Could you check a few things on this model? Use its own coordinates, in mm. Face numbers are marked on the shaded views. Give positions to 0.01 mm unless a question says otherwise; leave off trailing zeros. Order: outer loops, then holes, each group sorted by start corner. A loop starts at its lowest first (then second) coordinate and runs counter-clockwise, first axis right, second up.
(1) Imagine slicing it at A-A, the plane x = 1.75. Write out the boundary of the cut face in (y, z).
(2) If I drill on probe 1 along Z at (x, y) = (3.35, 0); probe 2 along Z at (x, y) = (2.1, 0); probe 3 along Z at (x, y) = (2.7, 0), over which ranges is the centre line in solid material (lowest first)?
(3) If we mould it in two halves opening along Z, with no side actions, what happens to the marked faces 1, 2 and 3? For each: released by +Z, released by -Z, zero draft, split by the parting line, or undercut.
(4) Will these pins go through, and if not, where does the flat tip stop? pin 1 (3 mm diameter, centred on x = 1, z = 5, fed in from +Y); pin 2 (1.5 mm diameter, centred on x = 2, y = -1.5, fed in from -Z); pin 3 (3 mm diameter, centred on x = 1, y = -7, fed in from -Z).
from build123d import *

# Parameters (mm, degrees)
F2_R     = 1.75
F3_DEPTH = 4


with BuildPart() as f1:
    # F0 (on Top) → F1 (revolve)
    with BuildSketch(Plane.XY):
        with BuildLine():
            Line((5, 10), (0, 10))
            ThreePointArc((0, 10), (-1.041182, 5.043677), (-1.5, 0))
            Line((-1.5, 0), (5, 0))
            Line((5, 0), (5, 3.291796))
            Line((5, 3.291796), (2.316718, 4.633437))
            Line((2.316718, 4.633437), (5, 10))
        make_face()
    revolve(axis=Axis((1.620585, 0, 0), (1, 0, 0)))

    # F2 (on face) → F3 (cut)
    with BuildSketch(Plane.YZ.offset(5)):
        Circle(F2_R)
    extrude(amount=-F3_DEPTH, mode=Mode.SUBTRACT)


solid = f1.part
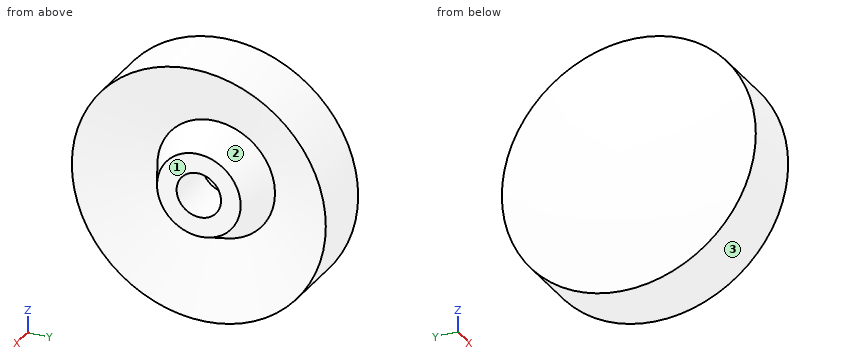
Answer block:
1. outline: circle Ø20 at (0, 0); hole circle Ø3.5 at (0, 0)
2. probe 1: z = -10 to -6.7, -4.12 to -1.75, 1.75 to 4.12, 6.7 to 10
2. probe 2: z = -10 to -1.75, 1.75 to 10
2. probe 3: z = -10 to -5.4, -4.44 to -1.75, 1.75 to 4.44, 5.4 to 10
3. face 1: zero draft
3. face 2: undercut
3. face 3: split by the parting line
4. pin 1: stops at y = 9.37
4. pin 2: stops at z = -9.97
4. pin 3: stops at z = -8.35
